```python
from build123d import *

# Parameters (mm, degrees)
F1_DEPTH = 25.4


with BuildPart() as f1:
    # F0 (on Right) → F1 (new body)
    with BuildSketch(Plane.YZ):
        with BuildLine():
            Line((0, -6.35), (0, 0))
            Line((0, 0), (-6.35, 0))
            Line((-6.35, 0), (-6.35, -3.81))
            ThreePointArc((-6.35, -3.81), (-4.553949, -4.553949), (-3.81, -6.35))
            Line((-3.81, -6.35), (0, -6.35))
        make_face()
        with BuildLine():
            Line((-6.35, -3.81), (-6.35, 0))
            Line((-6.35, 0), (-12.7, 0))
            Line((-12.7, 0), (-12.7, -6.35))
            Line((-12.7, -6.35), (-8.89, -6.35))
            ThreePointArc((-8.89, -6.35), (-8.146051, -4.553949), (-6.35, -3.81))
        make_face()
        with BuildLine():
            Line((-8.89, -6.35), (-12.7, -6.35))
            Line((-12.7, -6.35), (-12.7, -12.7))
            Line((-12.7, -12.7), (-6.35, -12.7))
            Line((-6.35, -12.7), (-6.35, -8.89))
            ThreePointArc((-6.35, -8.89), (-8.146051, -8.146051), (-8.89, -6.35))
        make_face()
        with BuildLine():
            Line((0, -12.7), (0, -6.35))
            Line((0, -6.35), (-3.81, -6.35))
            ThreePointArc((-3.81, -6.35), (-4.553949, -8.146051), (-6.35, -8.89))
            Line((-6.35, -8.89), (-6.35, -12.7))
            Line((-6.35, -12.7), (0, -12.7))
        make_face()
    extrude(amount=F1_DEPTH)


solid = f1.part
```
Here's how the part is built. I have some questions about the finished solid (model axes, mm). Round coordinates to 2 decimals unless told otherwise and drop trailing zeros. Order: outer loops, then holes, each group sorted by start corner. A loop starts at its lowest first (then second) coordinate and runs counter-clockwise, first axis right, second up. Notation, with made-up numbers: M 74.5,58.25 L 112.5,58.25 A19 ccw 112.5,86.25 Z; hole C 33.5,83.5 d6. An arc over 180 degrees is marked long. One line per question, with ' | ' between items.
1) I want a section at A-A, the plane z = -8.25. Write out the boundary of the cut face in (x, y).
Working result:
outline: M 0,-12.7 L 25.4,-12.7 L 25.4,-8.04 L 0,-8.04 Z; M 0,-4.66 L 25.4,-4.66 L 25.4,0 L 0,0 Z
2) I want a section at B-B, the plane y = -8. Write out the boundary of the cut face in (x, z), then the cut area to 3 significant figures.
Working result:
outline: M 0,-12.7 L 25.4,-12.7 L 25.4,-8.28 L 0,-8.28 Z; M 0,-4.42 L 25.4,-4.42 L 25.4,0 L 0,0 Z | area: 224 mm²
3) I need wall thicknesses on line 1 along Z through (x, y) = (18.25, -8); line 2 along Y through (x, z) = (1, -6); line 3 along Z through (x, y) = (18, -5.25). Which ranges of each line are inside material? Lowest first, please.
Working result:
line 1: -12.7 to -8.28, -4.42 to 0 | line 2: -12.7 to -8.87, -3.83 to 0 | line 3: -12.7 to -8.64, -4.06 to 0
4) I want a section at C-C, the plane x = 9.75. Write out the boundary of the cut face in (y, z).
Working result:
outline: M -12.7,-12.7 L 0,-12.7 L 0,0 L -12.7,0 Z; hole M -8.89,-6.35 A2.54 ccw -6.35,-8.89 A2.54 ccw -3.81,-6.35 A2.54 ccw -6.35,-3.81 A2.54 ccw Z
